Here's how the part is built. I have some questions about the finished solid (model axes, mm). Round coordinates to 2 decimals unless told otherwise and drop trailing zeros. Loops run counter-clockwise (first coordinate to the right, second up) from the corner with the lowest first, then second, coordinate; pieces in that order, holes last. Notation, with made-up numbers: M 30.25,51 L 81.25,51 A19 ccw 81.25,75 Z; hole C 83,-36.75 d11. An arc over 180 degrees is marked long. One line per question, with ' | ' between items. Start each with the question number.
Autodesk Inventor part; units mm, degrees
ref_plane "YZ Plane" through (0, 0, 0) normal (1, 0, 0) x (0, 1, 0)
ref_plane "XZ Plane" through (0, 0, 0) normal (0, 1, 0) x (-1, 0, 0)
ref_plane "XY Plane" through (0, 0, 0) normal (0, 0, 1) x (1, 0, 0)
sketch "Sketch1" plane through (0, 0, 0) normal (0, 0, 1) x (1, 0, 0)
  circle A0 centre (0, 0) radius 15
  circle A1 centre (77.2853, -100.6476) radius 15
  line L0 (0, 0) -> (77.2853, -100.6476) construction
  line L1 (4.6165, 51.4557) -> (140.1218, -125.0109) construction
  line L2 (-50.9034, 8.823) -> (49.7593, -122.2685) construction
  line L3 (11.1166, -71.9447) -> (66.6365, -29.312) construction
  line L4 (-50.9034, 8.823) -> (4.6165, 51.4557) construction
  line L5 (82.3144, -169.4001) -> (140.1218, -125.0109) construction
  line L6 (-50.9034, 8.823) -> (4.6165, 51.4557)
  line L7 (4.6165, 51.4557) -> (128.1887, -109.4706)
  line L8 (128.1887, -109.4706) -> (72.6688, -152.1033)
  line L9 (72.6688, -152.1033) -> (-50.9034, 8.823)
  point P0 (0, 0)
  dimension "d0" = 38
  dimension "d1" = 38
  dimension "d2" = 35
  dimension "d3" = 35
extrude "Extrusion1" add sketch "Sketch1" along normal blind 15
properties part number "gantry_y_holder"
1) Imagine slicing it at B-B (x = 0). Write out the boundary of the cut face in (y, z), then the cut area to 3 significant figures.
2) I'm going to push flat-ended pins straight in: pin 1 Ø6 at (y, z) = (-8, 5) entering from -X; pin 2 Ø2 at (x, z) = (-28, 9.5) entering from +Y; pin 3 Ø3 at (x, z) = (0, 6.5) entering from -Y. Where does each tip first touch, or does it pass through?
3) We'd pull the mould along X, two halves only. Please class faces 1 (the face through (-14.985, -0.66, 7.395)), 2 (the face through (91.593, -105.153, 7.395)), 3 (the face through (37, -49, 15)), 4 (the face through (11.75, -72.77, 7.4)): pulls with the +X half, pulls with the -X half, needs draft (parallel to the pull), parting line crosses it, or undercut.
4) Imagine slicing it at C-C (z = 11.75). Write out the boundary of the cut face in (x, y), then the cut area to 3 significant figures.
5) Imagine slicing it at A-A (y = 6). Write out the boundary of the cut face in (x, z), then the cut area to 3 significant figures.
6) Imagine slicing it at D-D (y = -124). Write out the boundary of the cut face in (x, z), then the cut area to 3 significant figures.
7) Please list where these lines run through material, in increasing order: L1, parallel to X at y = -6, z = 3.5; L2, parallel to Y at x = 0, z = 6.25; L3, parallel to Y at x = 84.5, z = 1.5. Write a range as from..to.
Results are:
1) outline: M -57.47,0 L -15,0 L -15,15 L -57.47,15 Z; M 15,0 L 47.91,0 L 47.91,15 L 15,15 Z | area: 1,130 mm²
2) pin 1: x = -40.29 | pin 2: y = 27.18 | pin 3: y = -59.42
3) face 1: undercut | face 2: undercut | face 3: needs draft | face 4: pulls with the -X half
4) outline: M -50.9,8.82 L 72.67,-152.1 L 128.19,-109.47 L 4.62,51.46 Z; hole C 0,0 d30; hole C 77.29,-100.65 d30 | area: 12,800 mm²
5) outline: M -48.74,0 L -13.75,0 L -13.75,15 L -48.74,15 Z; M 13.75,0 L 39.52,0 L 39.52,15 L 13.75,15 Z | area: 911 mm²
6) outline: M 51.09,0 L 109.27,0 L 109.27,15 L 51.09,15 Z | area: 873 mm²
7) L1: -39.52..-13.75, 13.75..48.74 | L2: -57.47..-15, 15..47.91 | L3: -143.02..-113.8, -87.5..-52.58
